Could you check a few things on this model? Use its own coordinates, in mm. Round coordinates to 2 decimals unless told otherwise and drop trailing zeros. Order: outer loops, then holes, each group sorted by start corner. A loop starts at its lowest first (then second) coordinate and runs counter-clockwise, first axis right, second up. Notation, with made-up numbers: (-35, 80) -> (8, 80) arc R18 ccw to (8, 106) -> close; hole circle Ø8 at (1.5, 66). An arc over 180 degrees is marked (long way). One line per question, with ' | ' between items.
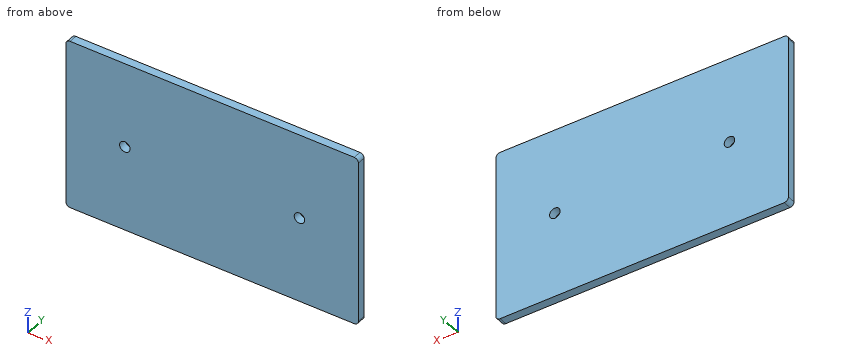
```python
from build123d import *

# Parameters (mm, degrees)
SKETCH1_W           = 88.9
SKETCH1_H           = 52.07
BOSS_EXTRUDE1_DEPTH = 2.54
FILLET1_R           = 1.27
SKETCH2_R           = 1.6
CUT_EXTRUDE1_DEPTH  = 7.62


with BuildPart() as part:
    # Sketch1 → Boss-Extrude1 (new body)
    with BuildSketch(Plane(origin=(0, 0, 0), x_dir=(1, 0, 0), z_dir=(0, 1, 0))):
        Rectangle(SKETCH1_W, SKETCH1_H)
    extrude(amount=BOSS_EXTRUDE1_DEPTH)

    # Fillet1
    fillet1_edges = [part.edges().sort_by_distance(p)[0] for p in [
        (-44.45, 1.27, -26.035),
        (44.45, 1.27, -26.035),
        (44.45, 1.27, 26.035),
        (-44.45, 1.27, 26.035),
    ]]
    fillet(fillet1_edges, radius=FILLET1_R)

    # Sketch2 → Cut-Extrude1 (cut)
    with BuildSketch(Plane(origin=(0, 2.54, 0), x_dir=(1, 0, 0), z_dir=(0, 1, 0))):
        with Locations((-26.543, 0)):
            Circle(SKETCH2_R)
        with Locations((26.543, 0)):
            Circle(SKETCH2_R)
    extrude(amount=-CUT_EXTRUDE1_DEPTH, mode=Mode.SUBTRACT)


solid = part.part
```
1. I want a section at A-A on z = 0. List the corners of the cut face in (x, y) for me.
From the geometry:
outline: (-44.45, 0) -> (-28.14, 0) -> (-28.14, 2.54) -> (-44.45, 2.54) -> close; (-24.94, 0) -> (24.94, 0) -> (24.94, 2.54) -> (-24.94, 2.54) -> close; (28.14, 0) -> (44.45, 0) -> (44.45, 2.54) -> (28.14, 2.54) -> close
2. I'm going to push a flat-ended pin straight in: pin 1 (2.5 mm diameter, centred on x = 26.543, z = 0, fed in from -Y). Where does the tip first touch, or does it pass through?
From the geometry:
pin 1: passes through
3. I need wall thicknesses on probe 1 along X at (y, z) = (0.5, 0); probe 2 along Z at (x, y) = (26.5, 1.1) (3 decimals); probe 3 along Z at (x, y) = (27.5, 1.7) (3 decimals). Which ranges of each line are inside material? Lowest first, please.
From the geometry:
probe 1: x = -44.45 to -28.14, -24.94 to 24.94, 28.14 to 44.45 | probe 2: z = -26.035 to -1.599, 1.599 to 26.035 | probe 3: z = -26.035 to -1.282, 1.282 to 26.035
